Build history of the part. All positions in model axes, mm. A direction names the side the tool comes from. Round coordinates to 2 decimals unless told otherwise and drop trailing zeros. Loops run counter-clockwise (first coordinate to the right, second up) from the corner with the lowest first, then second, coordinate; pieces in that order, holes last.
Autodesk Inventor part; units mm, degrees
ref_plane "YZ Plane" through (0, 0, 0) normal (1, 0, 0) x (0, 1, 0)
ref_plane "XZ Plane" through (0, 0, 0) normal (0, 1, 0) x (-1, 0, 0)
ref_plane "XY Plane" through (0, 0, 0) normal (0, 0, 1) x (1, 0, 0)
sketch "Esquisse1" plane through (0, 0, 0) normal (0, 0, 1) x (1, 0, 0)
  line L0 (-150.5839, 785.7) -> (150.5839, 785.7)
  arc A0 (150.5839, 785.7) -> (-150.5839, 785.7) centre (0, 0) ccw
  line L1 (-150.5839, 782.7) -> (150.5839, 782.7)
  line L2 (0, 797) -> (-150.5839, 797)
  arc A1 (150.5839, 782.7) -> (-150.5839, 782.7) centre (0, -3) ccw
  line L3 (-150.5839, 785.7) -> (-150.5839, 782.7)
  line L4 (150.5839, 785.7) -> (150.5839, 782.7)
  point P0 (0, 0)
  dimension "d4" = 785.7
  dimension "d8" = 3
  dimension "d9" = 14.3
extrude "Extrusion1" add sketch "Esquisse1" along normal blind 65 contours A0 L2 A1 L0 | L0 A1 L3 | A0 L0 A1 L2 | L0 L4 A1
ref_plane "Plan de construction1" through (-150.5839, 782.7, 65) normal (0, -1, 0) x (0, 0, -1)
sketch "Esquisse4" plane through (-150.5839, 782.7, 65) normal (0, -1, 0) x (0, 0, -1)
  line L0 (65, 301.1678) -> (65, 0)
  line L1 (30, 8) -> (65, 8)
  line L2 (65, 8) -> (65, 28)
  line L3 (65, 28) -> (30, 28)
  line L4 (30, 28) -> (30, 8)
  line L5 (65, 0) -> (0, 0)
  line L6 (65, 273.1678) -> (30, 273.1678)
  line L7 (30, 273.1678) -> (30, 293.1678)
  line L8 (30, 293.1678) -> (65, 293.1678)
  line L9 (65, 293.1678) -> (65, 273.1678)
  line L10 (65, 301.1678) -> (0, 301.1678)
  point P0 (65, 150.5839)
  point P1 (65, 8)
  dimension "d13" = 20
  dimension "d14" = 35
  dimension "d15" = 8
  dimension "d16" = 35
  dimension "d17" = 8
  dimension "d18" = 20
extrude "Extrusion2" add sketch "Esquisse4" against normal up to surface
sketch "Esquisse5" plane through (-150.5839, 782.7, 65) normal (0, -1, 0) x (1, 0, 0)
  line L0 (0, -65) -> (8, -65)
  line L1 (28, -30) -> (28, -65)
  line L2 (8, -65) -> (28, -65)
  line L3 (28, -65) -> (28, -30)
  line L4 (28, -30) -> (8, -30)
  line L5 (8, -30) -> (8, -65)
  line L6 (273.1678, -30) -> (293.1678, -30)
  line L7 (293.1678, -30) -> (293.1678, -65)
  line L8 (273.1678, -30) -> (293.1678, -30)
  line L9 (293.1678, -30) -> (293.1678, -65)
  line L10 (293.1678, -65) -> (273.1678, -65)
  line L11 (273.1678, -65) -> (273.1678, -30)
  point P0 (150.5839, -65)
extrude "Extrusion3" add sketch "Esquisse5" along normal blind 30
sketch "Esquisse9" plane through (0, 0, 65) normal (0, 0, 1) x (1, 0, 0)
  point P0 (0, 0)
sketch "Esquisse10" plane through (-150.5839, 782.7, 65) normal (0, -1, 0) x (0, 0, -1)
  line L0 (65, 301.1678) -> (0, 301.1678)
  line L1 (65, 301.1678) -> (68, 301.1678)
  line L2 (68, 301.1678) -> (68, 0)
  line L3 (68, 0) -> (65, 0)
  line L4 (65, 0) -> (65, 301.1678)
  point P0 (65, 150.5839)
  dimension "d81" = 3
extrude "Extrusion4" add sketch "Esquisse10" against normal blind 50
sketch "Esquisse11" plane through (-122.5839, 782.7, 0) normal (0, 0, 1) x (1, 0, 0)
  line L0 (-39.3889, 14.3) -> (313.6941, 14.3)
  line L1 (412.3411, 0) -> (-114.6772, 0)
  line L2 (273.1678, 0) -> (273.1678, 3)
  arc A0 (273.1678, 0) -> (-28, 0) centre (122.5839, -785.7) ccw
  line L3 (-28, 0) -> (273.1678, 0)
  point P0 (122.5839, -782.7)
  dimension "d84" = 14.3
extrude "Extrusion5" cut sketch "Esquisse11" against normal blind 10
sketch "Esquisse12" plane through (0, 0, 0) normal (0, 0, 1) x (1, 0, 0)
  line L0 (-152.2915, 801.4) -> (214.4689, 801.4)
  line L1 (288.3408, 782.7) -> (-228.7627, 782.7)
  line L2 (-154.8908, 815.7) -> (200.1728, 815.7)
  line L3 (150.5839, 785.7) -> (150.5839, 832.7)
  line L4 (-150.5839, 785.7) -> (-150.5839, 832.7)
  arc A0 (150.5839, 801.4) -> (-150.5839, 801.4) centre (0, 15.7) ccw
  line L5 (-150.5839, 801.4) -> (-150.5839, 832.7)
  line L6 (-150.5839, 832.7) -> (150.5839, 832.7)
  line L7 (150.5839, 832.7) -> (150.5839, 801.4)
  point P0 (0, 0)
  dimension "d87" = 18.7
  dimension "d88" = 14.3
extrude "Extrusion6" cut sketch "Esquisse12" against normal blind 10 contours L4 L2 A0 | A0 L2 L3 | L4 L6 L3 L2
sketch "Esquisse13" plane through (0, 0, 0) normal (0, 0, -1) x (-1, 0, 0)
  line L0 (142.5839, 784.1911) -> (142.5839, 752.7)
  line L1 (122.5839, 787.5525) -> (122.5839, 752.7)
  arc A0 (142.5839, 784.1911) -> (122.5839, 787.5525) centre (0, -3) ccw
  line L2 (142.5839, 784.1911) -> (142.5839, 752.7)
  line L3 (122.5839, 752.7) -> (142.5839, 752.7)
  line L4 (122.5839, 752.7) -> (122.5839, 787.5525)
  arc A1 (150.5839, 782.7) -> (-150.5839, 782.7) centre (0, -3) ccw
  arc A2 (-142.5839, 784.1911) -> (-122.5839, 787.5525) centre (0, -3) ccw
  line L5 (-122.5839, 787.5525) -> (-122.5839, 752.7)
  line L6 (-122.5839, 787.5525) -> (-122.5839, 752.7)
  line L7 (-142.5839, 752.7) -> (-122.5839, 752.7)
  line L8 (-122.5839, 752.7) -> (-142.5839, 752.7)
  line L9 (-142.5839, 784.1911) -> (-142.5839, 752.7)
  line L10 (-142.5839, 752.7) -> (-142.5839, 784.1911)
  arc A3 (-122.5839, 787.5525) -> (-142.5839, 784.1911) centre (0, -3) ccw
  point P0 (0, 0)
extrude "Extrusion7" add sketch "Esquisse13" along normal blind 3 contours L0 L3 L1 A0 | L5 L7 L9 A1
properties part number "arc_de_cercle"
(1) Probe line 1 (X direction, y = 756, z = 12); line 2 (Z direction, x = -74, y = 807.5); line 3 (Z direction, x = -132, y = 784.5). List the from-to ranges inside material, lowest first.
Responses:
line 1: x = -142.58 to -122.58, 122.58 to 142.58
line 2: z = -3 to 0
line 3: z = -3 to 35
(2) Pull direction X, two halves, no side cores. Call faces 1 (the face through (-2.121, 799.997, 32.045)), 2 (the face through (133, 752.7, 16)), 3 (the face through (2.121, 796.997, 31.476)): +X half, -X half, draft (parallel to the pull), parting line (faces both ways), or undercut.
Responses:
face 1: parting line
face 2: draft
face 3: undercut
(3) Slice it at C-C on x = 130.5. List the corners of the cut face in (y, z).
Responses:
outline: (752.7, -3) - (804.98, -3) - (804.98, 0) - (789.28, 0) - (789.28, 65) - (786.28, 65) - (786.28, 35) - (752.7, 35) - close
(4) Which spindle directions (+Z, -Z, +X, -X, +Y, -Y) get a long thin tool onto all of the face, cutting with end or side? Do faces 4 (the face through (-1, 798, 65)), 5 (the face through (-122.584, 770, 16)). Say none if no direction does.
Responses:
face 4: +Z, +X, -X, +Y, -Y
face 5: +Z, -Z, -Y
(5) Slice it at A-A on y = 765.5. List the corners of the cut face in (x, z), plus the area to 3 significant figures.
Responses:
outline: (-142.58, -3) - (-122.58, -3) - (-122.58, 35) - (-142.58, 35) - close; (122.58, -3) - (142.58, -3) - (142.58, 35) - (122.58, 35) - close
area: 1,520 mm2
(6) Pin check, flat tips, straight feed: P1, Ø2, axis at y = 778.5, z = 31, coming from the -X side; P2, Ø8, axis at y = 763.5, z = 11, coming from the +X side; P3, Ø22, axis at x = -136, y = 769.5, coming from the +Z side. Stop position of each tip, or through.
Responses:
P1: stops at x = -142.58
P2: stops at x = 142.58
P3: stops at z = 35
(7) Slice it at B-B on z = 6.5. List the corners of the cut face in (x, y).
Responses:
outline: (-150.58, 782.7) arc R800 cw to (-142.58, 784.19) - (-142.58, 752.7) - (-122.58, 752.7) - (-122.58, 787.55) arc R800 cw to (122.58, 787.55) - (122.58, 752.7) - (142.58, 752.7) - (142.58, 784.19) arc R800 cw to (150.58, 782.7) - (150.58, 785.7) arc R800 ccw to (-150.58, 785.7) - close
